```python
from build123d import *

# Parameters (mm, degrees)
BOSS_EXTRUDE1_DEPTH = 9.525
BOSS_EXTRUDE2_DEPTH = 9.525
FILLET1_R           = 15.875
SKETCH3_R           = 9.525
CUT_EXTRUDE1_DEPTH  = 587.481888574


with BuildPart() as part:
    # Sketch1 → Boss-Extrude1 (new body)
    with BuildSketch(Plane(origin=(0, 0, 0), x_dir=(1, 0, 0), z_dir=(0, 1, 0))):
        Polygon((461.512355724, 17.636671785), (558.8, 99.270698215), (558.8, 177.8), (228.6, 177.8), (228.6, -177.8), align=None)
    extrude(amount=BOSS_EXTRUDE1_DEPTH)

    # Sketch1_4 → Boss-Extrude2 (add)
    with BuildSketch(Plane(origin=(0, 0, 0), x_dir=(1, 0, 0), z_dir=(0, 1, 0))):
        Polygon((558.8, -177.8), (558.8, 99.270698215), (461.512355724, 17.636671785), (228.6, -177.8), align=None)
    extrude(amount=BOSS_EXTRUDE2_DEPTH)

    # Fillet1
    fillet1_edges = [part.edges().sort_by_distance(p)[0] for p in [
        (558.8, 4.7625, 177.8),
        (558.8, 4.7625, -177.8),
    ]]
    fillet(fillet1_edges, radius=FILLET1_R)

    # Sketch3 → Cut-Extrude1 (cut, through all)
    with BuildSketch(Plane.XZ):
        with Locations(Location((378.930433901, 124.074982269, 0), (0, 0, 270))):
            Circle(SKETCH3_R)
        with Locations(Location((448.729013979, 59.262015054, 0), (0, 0, 270))):
            Circle(SKETCH3_R)
        with BuildLine():
            ThreePointArc((510.787273965, 0), (525.902368362, -11.579080306), (511.547736048, 0.930344561))
            Line((511.547736048, 0.930344561), (512.549645575, 0))
            Line((512.549645575, 0), (510.787273965, 0))
        make_face()
        with Locations(Location((324.376240195, -74.656356713, 0), (0, 0, 270))):
            Circle(SKETCH3_R)
    extrude(amount=-CUT_EXTRUDE1_DEPTH, mode=Mode.SUBTRACT)


solid = part.part
```
Work out the finished part from the listing and answer in its coordinate system (mm). Give positions to 0.01 mm unless a question says otherwise; leave off trailing zeros. Order: outer loops, then holes, each group sorted by start corner. A loop starts at its lowest first (then second) coordinate and runs counter-clockwise, first axis right, second up. Notation, with made-up numbers: (-0.5, 24.5) -> (47.5, 24.5) arc R13 ccw to (47.5, 34.5) -> close; hole circle Ø3 at (36.25, 30). An arc over 180 degrees is marked (long way). Answer as CSV lines item,"result". Start each with the question number.
(1) Consider line 1 along Z through (x, y) = (325, 7.5); line 2 along Z through (x, y) = (320.5, 6); line 3 along X through (y, z) = (7.75, -12). Determine where each line is inside the solid, lowest interval first.
(2) Section B-B, the plane z = 63 is taken. Write down the section's boundary in (x, y) (3 decimals), plus the area to 3 significant figures.
(3) Section A-A, the plane x = 329 is taken. Write down the section's boundary in (y, z) (3 decimals), plus the area to 3 significant figures.
(4) For a pull along X with two mould halves and no side action, classify faces 1 (the flat face through (558.8, 5, 2)), 2 (the flat face through (391, 9.525, -2)), 3 (the cylindrical face through (451.59, 4.696, 50.177)) as released by +X, released by -X, zero draft, split by the parting line, or undercut.
Entries:
1,line 1,"-177.8 to -84.16, -65.15 to 177.8"
1,line 2,"-177.8 to -83.36, -65.96 to 177.8"
1,line 3,"228.6 to 511.52, 525.54 to 558.8"
2,outline,"(228.6, 0) -> (439.968, 0) -> (439.968, 9.525) -> (228.6, 9.525) -> close; (457.49, 0) -> (558.8, 0) -> (558.8, 9.525) -> (457.49, 9.525) -> close"
2,area,"2,980 mm²"
3,outline,"(0, -177.8) -> (9.525, -177.8) -> (9.525, -82.984) -> (0, -82.984) -> close; (0, -66.329) -> (9.525, -66.329) -> (9.525, 177.8) -> (0, 177.8) -> close"
3,area,"3,230 mm²"
4,face 1,"released by +X"
4,face 2,"zero draft"
4,face 3,"undercut"
